Check sheet for the modelled part. Datum: model origin and axes. Units: mm. Face numbers are marked on the shaded views. A direction names the side the tool comes from. Coordinates: 2 decimals unless noted, no trailing zeros. Loops run counter-clockwise (first coordinate to the right, second up) from the corner with the lowest first, then second, coordinate; pieces in that order, holes last. Notation, with made-up numbers: M 52.25,-11.75 L 87.25,-11.75 A15 cw 87.25,-4.75 Z; hole C -33,-4 d1. An arc over 180 degrees is marked long. Use CSV: the item, a comma, the result in double quotes. Start each with the question number.
(1) Section check C-C on x = 12.5. Record the cut outline in (y, z), and give its area (3 significant figures).
(2) Go/stop test with flat-tipped pins: pin 1 Ø1.1 at (x, z) = (-15, 16) entering from -Y; pin 2 Ø4.5 at (x, z) = (9.5, 20) entering from +Y; pin 3 Ø4 at (x, y) = (1.5, 6.5) entering from -Z; pin 4 Ø3 at (y, z) = (14, 19.5) entering from -X. Record where each tip stops, or that it passes through.
(3) Draft check along X on the marked faces 6, 7 and 8. Enter one of: pulls with the +X half, pulls with the -X half, needs draft (parallel to the pull), parting line crosses it, or undercut.
(4) Section check A-A on y = -1. Record the cut outline in (x, z).
(5) Section check D-D on y = -7. Record the cut outline in (x, z), and give its area (3 significant figures).
(6) Set-up check for the marked faces 1, 2, 3, 4 and 5: record each of +Z, -Z, +X, -X, +Y, -Y from which the full face is reachable in a straight line by a thin tool's end or side.
(7) Scan lines: line 1 (X direction, y = 0, z = 19.5); line 2 (Y direction, x = 14.5, z = 16.25); line 3 (Y direction, x = -16, z = 16). Record each from-to range of solid material in increasing order.
(8) Section check B-B on z = 20.75. Record the cut outline in (x, y).
from build123d import *

# Parameters (mm, degrees)
SKETCH1_W           = 45.72
SKETCH1_H           = 40.64
BOSS_EXTRUDE1_DEPTH = 13.97
SKETCH2_W           = 7.220890655
SKETCH2_H           = 24.390563991
SKETCH2_W_2         = 12.141793916
SKETCH2_H_2         = 6.044152918
SKETCH2_W_3         = 7.434842971
SKETCH2_H_3         = 13.104579336
SKETCH2_W_4         = 13.960388599
SKETCH2_H_4         = 6.097640998
BOSS_EXTRUDE2_DEPTH = 8.89
SKETCH3_W           = 18.292922993
SKETCH3_H           = 7.595307208
BOSS_EXTRUDE3_DEPTH = 8.89
SKETCH4_W           = 14.869685941
SKETCH4_H           = 6.311593313
BOSS_EXTRUDE4_DEPTH = 3.81


with BuildPart() as part:
    # Sketch1 → Boss-Extrude1 (new body)
    with BuildSketch(Plane.XY):
        Rectangle(SKETCH1_W, SKETCH1_H)
    extrude(amount=BOSS_EXTRUDE1_DEPTH)

    # Sketch2 → Boss-Extrude2 (add)
    with BuildSketch(Plane.XY.offset(13.97)):
        with Locations((-17.517345848, 3.663933406)):
            Rectangle(SKETCH2_W, SKETCH2_H)
        with Locations((11.152264456, 15.137126336)):
            Rectangle(SKETCH2_W_2, SKETCH2_H_2)
        with Locations((17.94525048, 2.139523157)):
            Rectangle(SKETCH2_W_3, SKETCH2_H_3)
        with Locations((10.724359825, -13.45225185)):
            Rectangle(SKETCH2_W_4, SKETCH2_H_4)
    extrude(amount=BOSS_EXTRUDE2_DEPTH)

    # Sketch3 → Boss-Extrude3 (add)
    with BuildSketch(Plane.XY.offset(13.97)):
        with Locations((-1.123249658, 1.203481776)):
            Rectangle(SKETCH3_W, SKETCH3_H)
    extrude(amount=BOSS_EXTRUDE3_DEPTH)

    # Sketch4 → Boss-Extrude4 (add)
    with BuildSketch(Plane.XY.offset(13.97)):
        with Locations((-11.927841601, -14.361549191)):
            Rectangle(SKETCH4_W, SKETCH4_H)
    extrude(amount=BOSS_EXTRUDE4_DEPTH)


solid = part.part
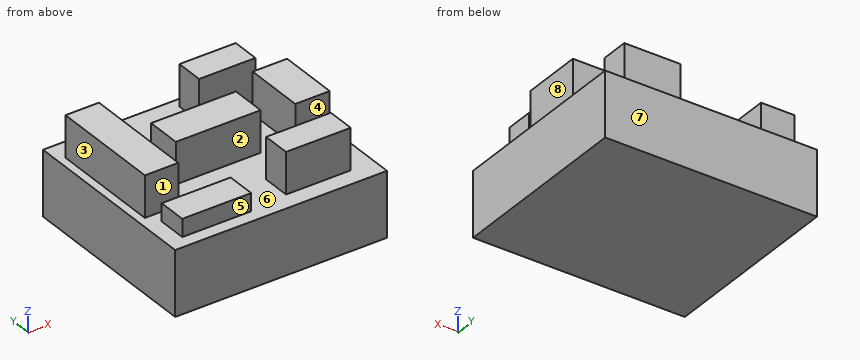
Outcome:
1,outline,"M -20.32,0 L 20.32,0 L 20.32,13.97 L 18.16,13.97 L 18.16,22.86 L 12.12,22.86 L 12.12,13.97 L -10.4,13.97 L -10.4,22.86 L -16.5,22.86 L -16.5,13.97 L -20.32,13.97 Z"
1,area,"676 mm²"
2,pin 1,"stops at y = -17.52"
2,pin 2,"stops at y = 18.16"
2,pin 3,"stops at z = 0"
2,pin 4,"stops at x = -21.13"
3,face 6,"undercut"
3,face 7,"needs draft"
3,face 8,"pulls with the +X half"
4,outline,"M -22.86,0 L 22.86,0 L 22.86,13.97 L 21.66,13.97 L 21.66,22.86 L 14.23,22.86 L 14.23,13.97 L 8.02,13.97 L 8.02,22.86 L -10.27,22.86 L -10.27,13.97 L -13.91,13.97 L -13.91,22.86 L -21.13,22.86 L -21.13,13.97 L -22.86,13.97 Z"
5,outline,"M -22.86,0 L 22.86,0 L 22.86,13.97 L -13.91,13.97 L -13.91,22.86 L -21.13,22.86 L -21.13,13.97 L -22.86,13.97 Z"
5,area,"703 mm²"
6,face 1,"+Z, +X, -X"
6,face 2,"+Z"
6,face 3,"+Z, -X, +Y, -Y"
6,face 4,"+Z, +X"
6,face 5,"+Z, +X, -X, -Y"
7,line 1,"x = -21.13 to -13.91, -10.27 to 8.02, 14.23 to 21.66"
7,line 2,"y = -16.5 to -10.4, -4.41 to 8.69, 12.12 to 18.16"
7,line 3,"y = -17.52 to -11.21, -8.53 to 15.86"
8,outline,"M -21.13,-8.53 L -13.91,-8.53 L -13.91,15.86 L -21.13,15.86 Z; M -10.27,-2.59 L 8.02,-2.59 L 8.02,5 L -10.27,5 Z; M 3.74,-16.5 L 17.7,-16.5 L 17.7,-10.4 L 3.74,-10.4 Z; M 5.08,12.12 L 17.22,12.12 L 17.22,18.16 L 5.08,18.16 Z; M 14.23,-4.41 L 21.66,-4.41 L 21.66,8.69 L 14.23,8.69 Z"
